```python
from build123d import *

# Parameters (mm, degrees)
SKETCH1_R           = 4.5
BOSS_EXTRUDE1_DEPTH = 10
SHELL1_T            = -1
FILLET1_R           = 1


with BuildPart() as part:
    # Sketch1 → Boss-Extrude1 (new body)
    with BuildSketch(Plane(origin=(0, 0, 0), x_dir=(1, 0, 0), z_dir=(0, 1, 0))):
        with Locations(Location((0, 0, 0), (0, 0, 270))):
            Circle(SKETCH1_R)
    extrude(amount=BOSS_EXTRUDE1_DEPTH)

    # Shell1
    shell1_openings = [part.faces().sort_by_distance(p)[0] for p in [
        (0, 10, 0),
    ]]
    offset(amount=SHELL1_T, openings=shell1_openings, kind=Kind.INTERSECTION)

    # Sketch4 → Cut-Revolve1 (revolve, cut)
    with BuildSketch(Plane.XY):
        with BuildLine():
            Line((0, 3.5), (0, -1.5))
            ThreePointArc((0, -1.5), (2.5, 1), (0, 3.5))
        make_face()
    revolve(axis=Axis((0, 3.5, 0), (0, -1, 0)), mode=Mode.SUBTRACT)

    # Fillet1
    fillet1_edges = [part.edges().sort_by_distance(p)[0] for p in [
        (0, 0, -4.5),
    ]]
    fillet(fillet1_edges, radius=FILLET1_R)


solid = part.part
```
Geometry: final body of the model. Coordinates: model frame, mm. Round coordinates to 2 decimals unless told otherwise and drop trailing zeros. Order: outer loops, then holes, each group sorted by start corner. A loop starts at its lowest first (then second) coordinate and runs counter-clockwise, first axis right, second up. Notation, with made-up numbers: (-10.75, 27) -> (10.25, 27) arc R10 ccw to (10.25, 44) -> close; hole circle Ø4 at (-11, 85). An arc over 180 degrees is marked (long way). Write each question's results on one line, items separated by ' | '.
Q1. Section query B-B (x = 0). Output: boundary loops of the cut face in (y, z), and give its area (3 significant figures).
Response values:
outline: (0, -3.5) arc R1 ccw to (1, -4.5) -> (10, -4.5) -> (10, -3.5) -> (1, -3.5) -> (1, -2.5) arc R2.5 cw to (0, -2.29) -> close; (0, 2.29) arc R2.5 cw to (1, 2.5) -> (1, 3.5) -> (10, 3.5) -> (10, 4.5) -> (1, 4.5) arc R1 ccw to (0, 3.5) -> close | area: 21.7 mm²
Q2. Pin query (flat end, axial travel): pin 1 Ø1 at (x, y) = (2.5, 7) entering from -Z; pin 2 Ø5 at (x, y) = (3, 8.5) entering from -Z; pin 3 Ø1.5 at (x, y) = (-2.5, 7) entering from -Z. Return the tip coordinate at first contact, or that it passes through.
Response values:
pin 1: z = -4.03 | pin 2: z = -4.47 | pin 3: z = -4.15
Q3. Ray query, line 1 along X through (y, z) = (4, 0); line 2 along X through (y, z) = (8.25, -3); line 3 along Z through (x, y) = (-1.75, 0.75). Return the intervals inside material, ascending.
Response values:
line 1: -4.5 to -3.5, 3.5 to 4.5 | line 2: -3.35 to -1.8, 1.8 to 3.35 | line 3: -4.11 to -1.77, 1.77 to 4.11
Q4. Pull-direction query (X, two-part tool) for faces 1 (the face through (1.352, 5.437, 4.292)), 2 (the face through (-2, 1, 2)), 3 (the face through (-4, 10, 0)); classes: released by +X, released by -X, zero draft, split by the parting line, or undercut.
Response values:
face 1: split by the parting line | face 2: undercut | face 3: zero draft
Q5. Section query C-C (y = 2). Output: boundary loops of the cut face in (x, z).
Response values:
outline: circle Ø9 at (0, 0); hole circle Ø7 at (0, 0)
Q6. Section query A-A (z = 0). Output: boundary loops of the cut face in (x, y), and give its area (3 significant figures).
Response values:
outline: (-4.5, 1) arc R1 ccw to (-3.5, 0) -> (-2.29, 0) arc R2.5 cw to (-2.5, 1) -> (-3.5, 1) -> (-3.5, 10) -> (-4.5, 10) -> close; (2.29, 0) -> (3.5, 0) arc R1 ccw to (4.5, 1) -> (4.5, 10) -> (3.5, 10) -> (3.5, 1) -> (2.5, 1) arc R2.5 cw to start | area: 21.7 mm²
